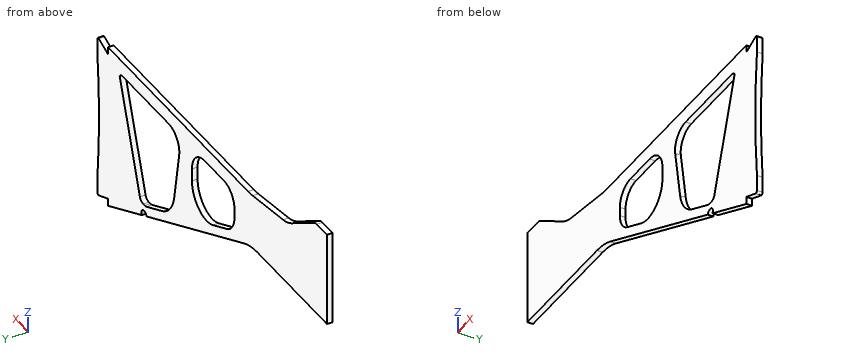
```python
from build123d import *

# Parameters (mm, degrees)
F1_DEPTH = 3


with BuildPart() as f1:
    # F0 (on Front) → F1 (new body)
    with BuildSketch(Plane.XZ):
        with BuildLine():
            Line((9.547373, 0), (0, 0))
            Line((0, 0), (0, -50.61))
            Line((0, -50.61), (65.50128, -50.61))
            ThreePointArc((65.50128, -50.61), (71.852686, -51.290047), (77.916141, -53.299357))
            Line((77.916141, -53.299357), (169.617761, -94.98504))
            ThreePointArc((169.617761, -94.98504), (172.383668, -93.272901), (174.5, -95.743285))
            ThreePointArc((174.5, -95.743285), (174.407699, -96.416327), (174.137612, -97.039671))
            Line((174.137612, -97.039671), (205.947947, -111.5))
            Line((205.947947, -111.5), (205.947947, -107.5))
            Line((205.947947, -107.5), (214.576557, -110.951444))
            ThreePointArc((214.576557, -110.951444), (215.508576, -110.851034), (215.947947, -110.022967))
            Line((215.947947, -110.022967), (215.947947, -101.5))
            ThreePointArc((215.947947, -101.5), (214.419617, -66.5), (215.947947, -31.5))
            Line((215.947947, -31.5), (215.947947, -22.977033))
            ThreePointArc((215.947947, -22.977033), (215.508576, -22.148966), (214.576557, -22.048556))
            Line((214.576557, -22.048556), (205.947947, -25.5))
            Line((205.947947, -25.5), (205.947947, -21.5))
            Line((205.947947, -21.5), (74.132034, -21.5))
            ThreePointArc((74.132034, -21.5), (72.005364, -21.424526), (69.889394, -21.198485))
            Line((69.889394, -21.198485), (41.25714, -17.108163))
            ThreePointArc((41.25714, -17.108163), (37.158324, -16.07119), (33.369079, -14.195761))
            Line((33.369079, -14.195761), (12.226495, -0.778353))
            ThreePointArc((12.226495, -0.778353), (10.942322, -0.19853), (9.547373, 0))
        make_face()
        with BuildLine():
            ThreePointArc((139.015857, -41.198191), (141.222671, -33.057249), (148.870609, -29.5))
            Line((148.870609, -29.5), (192.401924, -29.5))
            ThreePointArc((192.401924, -29.5), (193.901924, -29.901924), (195, -31))
            Line((195, -31), (175.934504, -87.76478))
            ThreePointArc((175.934504, -87.76478), (174.690897, -89.347155), (172.727083, -89.787502))
            ThreePointArc((172.727083, -89.787502), (172.014742, -89.743303), (171.302191, -89.784002))
            ThreePointArc((171.302191, -89.784002), (170.490013, -89.768373), (169.711801, -89.535424))
            Line((169.711801, -89.535424), (154.550645, -82.643472))
            ThreePointArc((154.550645, -82.643472), (147.348811, -76.674589), (143.648817, -68.083663))
            Line((143.648817, -68.083663), (139.015857, -41.198191))
        make_face(mode=Mode.SUBTRACT)
        with BuildLine():
            ThreePointArc((87, -39.5), (89.928932, -32.428932), (97, -29.5))
            Line((97, -29.5), (115, -29.5))
            ThreePointArc((115, -29.5), (123.485281, -33.014719), (127, -41.5))
            Line((127, -41.5), (127, -48.376778))
            ThreePointArc((127, -48.376778), (120.579234, -60.147726), (107.206398, -61.121745))
            Line((107.206398, -61.121745), (94.034056, -55.133867))
            ThreePointArc((94.034056, -55.133867), (88.910616, -50.706096), (87, -44.20961))
            Line((87, -44.20961), (87, -39.5))
        make_face(mode=Mode.SUBTRACT)
    extrude(amount=F1_DEPTH)


solid = f1.part
```
Part model, mm, in its own coordinate system. Round coordinates to 2 decimals unless told otherwise and drop trailing zeros. Loops run counter-clockwise (first coordinate to the right, second up) from the corner with the lowest first, then second, coordinate; pieces in that order, holes last. Notation, with made-up numbers: (-19, 24) -> (8, 24) arc R15 cw to (8, 34) -> close; hole circle Ø10 at (33.25, 71.25). An arc over 180 degrees is marked (long way). Use one line per item in the form item = value. Start each with the question number.
Item 1: Band-saw the part on D-D (x = 50.5). List the corners of the cut face in (y, z), plus the area to 3 significant figures.
Item 2: Drill centre lines: line 1 along X through (y, z) = (-2.85, -44.5); line 2 along X through (y, z) = (-1.5, -58); line 3 along X through (y, z) = (-1.05, -62.5). Where is each one in solid material? Low to high.
Item 3: Band-saw the part on B-B (z = -78). List the corners of the cut face in (x, y).
Item 4: Band-saw the part on C-C (y = -0.5). Give the number of separate pieces and of enclosed holes in the cut face, plus the area to 3 significant figures.
Item 5: Drop flat-ended pins along their axis: pin 1 Ø0.9 at (x, y) = (132, -1) entering from +Z; pin 2 Ø0.9 at (x, y) = (102.5, -1) entering from -Z; pin 3 Ø1.5 at (x, y) = (166, -2) entering from -Z. Give the stop position or say it passes through.
Item 6: Band-saw the part on A-A (x = 158.5). List the corners of the cut face in (y, z), plus the area to 3 significant figures.
Data:
q1.outline = (-3, -50.61) -> (0, -50.61) -> (0, -18.43) -> (-3, -18.43) -> close
q1.area = 96.5 mm^2
q2.line_1 = 0 to 87, 127 to 139.58, 190.47 to 215.02
q2.line_2 = 88.26 to 100.34, 123.17 to 141.91, 185.93 to 214.51
q2.line_3 = 98.16 to 142.69, 184.42 to 214.44
q3.outline = (132.25, -3) -> (148.43, -3) -> (148.43, 0) -> (132.25, 0) -> close; (179.21, -3) -> (214.58, -3) -> (214.58, 0) -> (179.21, 0) -> close
q4.separate_pieces = 1
q4.enclosed_holes = 2
q4.area = 8,010 mm^2
q5.pin_1 = -21.5
q5.pin_2 = -64.68
q5.pin_3 = -93.68
q6.outline = (-3, -89.93) -> (0, -89.93) -> (0, -84.44) -> (-3, -84.44) -> close; (-3, -29.5) -> (0, -29.5) -> (0, -21.5) -> (-3, -21.5) -> close
q6.area = 40.5 mm^2
